from build123d import *

# Parameters (mm, degrees)
F0_R     = 13
F0_R_2   = 10
F1_DEPTH = 2
F0_R_3   = 8.5
F2_DEPTH = 4
F3_DEPTH = 2


with BuildPart() as f1:
    # F0 (on Front) → F1 (new body)
    with BuildSketch(Plane.XZ):
        Circle(F0_R)
        Circle(F0_R_2, mode=Mode.SUBTRACT)
    extrude(amount=-F1_DEPTH)

    # F0 (on Front) → F2 (join)
    with BuildSketch(Plane.XZ):
        Circle(F0_R_2)
        Circle(F0_R_3, mode=Mode.SUBTRACT)
    extrude(amount=-F2_DEPTH)

    # F0 (on Front) → F3 (join)
    with BuildSketch(Plane.XZ):
        Circle(F0_R_3)
    extrude(amount=-F3_DEPTH)


solid = f1.part
The model under review builds one solid part; all positions refer to its coordinate system, in mm. A direction names the side the tool comes from. Coordinates: 2 decimals unless noted, no trailing zeros. Loops run counter-clockwise (first coordinate to the right, second up) from the corner with the lowest first, then second, coordinate; pieces in that order, holes last. Notation, with made-up numbers: M 0,16.25 L 32,16.25 A29 ccw 32,42.25 Z; hole C -9.75,67 d7. An arc over 180 degrees is marked long. Put each result on its own line as item: value. Start each with the question number.
Q1. Add section B-B (z = 0). Write out the cut boundary in (x, y).
Q2. Add section D-D (z = -9.25). Write out the cut boundary in (x, y), and give its area (3 significant figures).
Q3. Add section C-C (y = 3.3). Write out the cut boundary in (x, z).
Q4. Add section A-A (x = 0). Write out the cut boundary in (y, z), and give its area (3 significant figures).
Q5. For faces 4 (the flat face through (-4.5, 4, -7.4)), 5 (the cylindrical face through (-2.17, 2.99, -9.76)), list the 3-axis set-ups (+Z, -Z, +X, -X, +Y, -Y) from which the entire face can be reached by the end or side of a thin tool; tool diameter is ignored.
Q6. Clearance check with flat-ended pins moving along their axes: pin 1 (3 mm diameter, centred on x = 4.5, z = 2.5, fed in from +Y); pin 2 (1.5 mm diameter, centred on y = 2, z = 5, fed in from -X); pin 3 (1.5 mm diameter, centred on x = -3, y = 3, fed in from +Z). State where each tip first meets the part, or that it passes through.
Q7. Wall thickness on line 1 (Z direction, x = 0, y = 2.7); line 2 (Z direction, x = 2.5, y = 2.45); line 3 (Y direction, x = 10.75, z = 3.5): over which ranges is each line inside the solid? List them lowest first.
Q8. The part is to be moulded in two halves that separate along X. For faces 1 (the flat face through (0, 0, 0)), 2 (the cylindrical face through (-10.316, 0.986, -7.91)), 3 (the flat face through (0, 2, 0)), say which applies: +X half, -X half, draft (parallel to the pull), parting line (faces both ways), or undercut.
Answers:
1. outline: M -13,0 L 13,0 L 13,2 L 10,2 L 10,4 L 8.5,4 L 8.5,2 L -8.5,2 L -8.5,4 L -10,4 L -10,2 L -13,2 Z
2. outline: M -9.13,0 L 9.13,0 L 9.13,2 L 3.8,2 L 3.8,4 L -3.8,4 L -3.8,2 L -9.13,2 Z
2. area: 51.7 mm^2
3. outline: C 0,0 d20; hole C 0,0 d17
4. outline: M 0,-13 L 2,-13 L 2,-10 L 4,-10 L 4,-8.5 L 2,-8.5 L 2,8.5 L 4,8.5 L 4,10 L 2,10 L 2,13 L 0,13 Z
4. area: 58.0 mm^2
5. face 4: +Z, -Z, +X, -X, +Y
5. face 5: +Y
6. pin 1: stops at y = 2
6. pin 2: stops at x = -12.29
6. pin 3: stops at z = 9.74
7. line 1: z = -10 to -8.5, 8.5 to 10
7. line 2: z = -9.68 to -8.12, 8.12 to 9.68
7. line 3: y = 0 to 2
8. face 1: draft
8. face 2: parting line
8. face 3: undercut
